Autodesk Inventor part; units mm, degrees
ref_plane "Work Plane1" through (0, 0, 103) normal (0, 0, 1) x (1, 0, 0)
ref_plane "Work Plane2" through (0, 0, 5) normal (0, 0, -1) x (-1, 0, 0)
ref_plane "YZ Plane" through (0, 0, 0) normal (1, 0, 0) x (0, 1, 0)
sketch "Sketch1" plane through (0, 0, 0) normal (0, 0, 1) x (1, 0, 0)
  line L0 (0, 16) -> (0, 5)
  line L1 (5, 0) -> (195, 0)
  line L2 (200, 5) -> (200, 16)
  arc A0 (0, 5) -> (5, 0) centre (5, 5) ccw
  arc A1 (195, 0) -> (200, 5) centre (195, 5) ccw
  line L3 (2, 16) -> (2, 5)
  arc A2 (2, 5) -> (5, 2) centre (5, 5) ccw
  line L4 (5, 2) -> (195, 2)
  arc A3 (195, 2) -> (198, 5) centre (195, 5) ccw
  line L5 (198, 5) -> (198, 16)
  line L6 (0, 16) -> (2, 16)
  line L7 (198, 16) -> (200, 16)
  point P0 (0, 0)
  dimension "fillet2" = 5
  dimension "thickness2" = 2
  dimension "caseBottomWidth2" = 200
  dimension "caseBottomHeight2" = 16
extrude "Extrusion1" add sketch "Sketch1" along normal blind 108
ref_plane "Work Plane1" through (0, 0, 103) normal (0, 0, 1) x (1, 0, 0)
sketch "Sketch3" plane through (0, 0, 103) normal (0, 0, 1) x (1, 0, 0)
  line L0 (2, 16) -> (1, 16)
  line L1 (2, 16) -> (2, 5)
  line L2 (1, 16) -> (1, 5)
  line L3 (195, 2) -> (5, 2)
  line L4 (195, 2) -> (5, 2)
  line L5 (198, 16) -> (198, 5)
  line L6 (198, 16) -> (198, 5)
  line L7 (198, 16) -> (199, 16)
  line L8 (199, 16) -> (199, 5)
  line L9 (5, 1) -> (195, 1)
  arc A0 (2, 5) -> (5, 2) centre (5, 5) ccw
  arc A1 (195, 2) -> (198, 5) centre (195, 5) ccw
  arc A2 (1, 5) -> (5, 1) centre (5, 5) ccw
  arc A3 (195, 1) -> (199, 5) centre (195, 5) ccw
  point P0 (0, 0)
  dimension "d8" = 1
  dimension "d9" = 1
  dimension "d10" = 1
  dimension "filletInner2" = 3
  dimension "filletMid2" = 4
extrude "Extrusion2" cut sketch "Sketch3" against normal blind 2
ref_plane "Work Plane2" through (0, 0, 5) normal (0, 0, -1) x (-1, 0, 0)
sketch "Sketch5" plane through (0, 0, 5) normal (0, 0, -1) x (-1, 0, 0)
  line L0 (-200, 16) -> (-198, 16)
  line L1 (-198, 16) -> (-198, 5)
  line L2 (-199, 16) -> (-199, 5)
  line L3 (-2, 5) -> (-2, 16)
  line L4 (-2, 16) -> (-2, 5)
  line L5 (-2, 16) -> (0, 16)
  line L6 (-1, 16) -> (-1, 5)
  line L7 (-195, 2) -> (-5, 2)
  line L8 (-195, 1) -> (-5, 1)
  line L9 (-195, 2) -> (-5, 2)
  arc A0 (-198, 5) -> (-195, 2) centre (-195, 5) ccw
  arc A1 (-5, 2) -> (-2, 5) centre (-5, 5) ccw
  arc A2 (-199, 5) -> (-195, 1) centre (-195, 5) ccw
  arc A3 (-5, 1) -> (-1, 5) centre (-5, 5) ccw
  point P0 (0, 0)
  dimension "d21" = 1
  dimension "d22" = 3
  dimension "d23" = 4
extrude "Extrusion4" cut sketch "Sketch5" against normal blind 2
sketch "Sketch7" plane through (0, 0, 108) normal (0, 0, 1) x (1, 0, 0)
  line L0 (2, 16) -> (0, 16)
  line L1 (2, 16) -> (1, 16)
  line L2 (1, 16) -> (1, 15)
  line L3 (1, 15) -> (2, 15)
  line L4 (2, 15) -> (2, 16)
  line L5 (199, 5) -> (199, 16)
  line L6 (198, 16) -> (198, 5)
  line L7 (199, 16) -> (198, 16)
  line L8 (198, 16) -> (198, 15)
  line L9 (198, 15) -> (199, 15)
  line L10 (199, 15) -> (199, 16)
  point P0 (0, 0)
  dimension "d28" = 1
  dimension "d29" = 1
extrude "Extrusion6" cut sketch "Sketch7" against normal through all
sketch "Sketch8" plane through (5, 2, 101) normal (0, 1, 0) x (1, 0, 0)
  circle A0 centre (4, 76) radius 4
  line L0 (-5, 101) -> (-5, -7)
  line L1 (190, 101) -> (0, 101)
  circle A1 centre (184, 76) radius 4
  circle A2 centre (4, 13) radius 4
  circle A3 centre (184, 13) radius 4
  dimension "d32" = 9
  dimension "d33" = 25
  dimension "d34" = 8
  dimension "d37" = 180
  dimension "d40" = 63
extrude "Extrusion7" add sketch "Sketch8" along normal blind 13
sketch "Sketch9" plane through (9, 15, 88) normal (0, 1, 0) x (1, 0, 0)
  circle A0 centre (0, 63) radius 4
  circle A1 centre (0, 63) radius 1.7
  circle A2 centre (0, 0) radius 1.7
  circle A3 centre (180, 0) radius 1.7
  circle A4 centre (180, 63) radius 4
  circle A5 centre (180, 63) radius 1.7
  circle A6 centre (180, 0) radius 4
  circle A7 centre (0, 0) radius 4
  point P0 (-9, 88)
  dimension "d45" = 3.4
extrude "Extrusion8" cut sketch "Sketch9" against normal blind 12 contours A1 | A2 | A3 | A5
equation "\"fillet2\" = fillet"
equation "\"thickness2\" = thickness"
equation "\"caseBottomWidth2\" = caseBottomWidth"
equation "\"caseBottomHeight2\" = caseBottomHeight"
equation "\"caseBottomDepth2\" = caseBottomDepth"
equation "\"d8\" = 0.5 * thickness2"
equation "\"d9\" = 0.5 * thickness2"
equation "\"d10\" = 0.5 * thickness2"
equation "\"filletInner2\" = filletInner"
equation "\"filletMid2\" = filletMid"
equation "\"d13\" = thickness2"
equation "\"d21\" = 0.5 * thickness2"
equation "\"d22\" = filletInner2"
equation "\"d23\" = filletMid2"
equation "\"d24\" = thickness2"
equation "\"d28\" = lipHeight"
equation "\"d29\" = 0.5 * thickness"
equation "\"d32\" = caseJoinOffsetFromSide"
equation "\"d33\" = caseJoinOffsetFromBack"
equation "\"d34\" = caseJoinDiameter"
equation "\"d37\" = caseJoinSpacingLeftRight"
equation "\"d40\" = caseJoinSpacingFrontBack"
equation "\"d43\" = caseBottomHeight2 - 1.5 * thickness"
equation "\"d45\" = holeDiameter"
equation "\"d46\" = caseBottomHeight2 - 2 * thickness"
equation "\"frontBackOffset2\" = frontBackOffset"
equation "\"d15\" = frontBackOffset2"
properties part number "case-bottom"
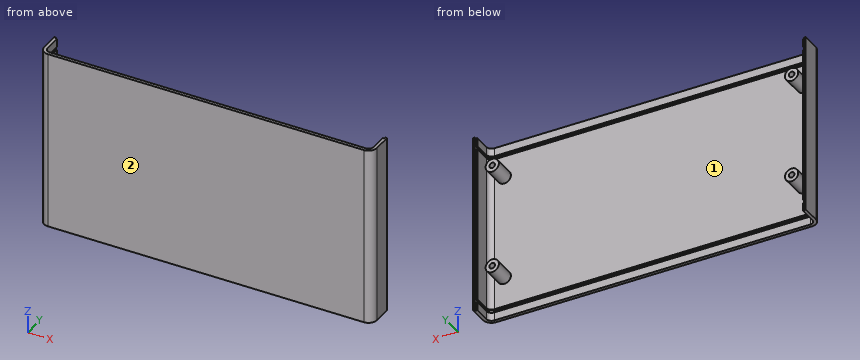
Source: CAD feature listing. Evaluate the final solid. Frame: model axes, mm. Face numbers are marked on the shaded views. Give positions to 0.01 mm unless a question says otherwise; leave off trailing zeros. Write each loop counter-clockwise with the first axis right and the second up, starting at its lowest first coordinate (ties: lowest second). Pieces come first, ordered by that corner, then holes.
1. First-contact query: pin 1 (3 mm diameter, centred on x = 141, z = 14.5, fed in from +Y); pin 2 (4.5 mm diameter, centred on x = 9, z = 25, fed in from +Y). Flat tips, straight axial feed; report the tip coordinate or a pass-through.
2. Section query B-B (z = 36). Return the cut outline in (x, y).
3. Pull-direction query (X, two-part tool) for the marked faces 1 and 2; classes: +X half, -X half, draft (parallel to the pull), parting line (faces both ways), or undercut.
4. Material intervals for line 1 along Z through (x, y) = (9, 7); line 2 along Z through (x, y) = (122.5, 1.5); line 3 along X through (y, z) = (9.25, 25), sorted ascending.
5. Section query A-A (y = 7.25). Count the separate pieces of the cut face and the enclosed holes in it, then the cut area to 3 significant figures.
6. Section query C-C (x = 64). Return the cut outline in (y, z), then the cut area to 3 significant figures.
Output values:
1. pin 1: stops at y = 2
1. pin 2: stops at y = 15
2. outline: (0, 5) arc R5 ccw to (5, 0) - (195, 0) arc R5 ccw to (200, 5) - (200, 16) - (199, 16) - (199, 15) - (198, 15) - (198, 5) arc R3 cw to (195, 2) - (5, 2) arc R3 cw to (2, 5) - (2, 15) - (1, 15) - (1, 16) - (0, 16) - close
3. face 1: undercut
3. face 2: draft
4. line 1: z = 21 to 23.3, 26.7 to 29, 84 to 86.3, 89.7 to 92
4. line 2: z = 0 to 5, 7 to 101, 103 to 108
4. line 3: x = 0 to 2, 5 to 7.3, 10.7 to 13, 185 to 187.3, 190.7 to 193, 198 to 200
5. separate pieces: 6
5. enclosed holes: 4
5. area: 589 mm2
6. outline: (0, 0) - (2, 0) - (2, 5) - (1, 5) - (1, 7) - (2, 7) - (2, 101) - (1, 101) - (1, 103) - (2, 103) - (2, 108) - (0, 108) - close
6. area: 212 mm2
